Design review of the part built by this model. Coordinates are the model's own, in mm. A direction names the side the tool comes from. Coordinates: 2 decimals unless noted, no trailing zeros. Loops run counter-clockwise (first coordinate to the right, second up) from the corner with the lowest first, then second, coordinate; pieces in that order, holes last. Notation, with made-up numbers: (53, 17) - (73, 17) arc R26 ccw to (73, 36) - close; hole circle Ø3 at (12.25, 13.25). An arc over 180 degrees is marked (long way). Answer in a Markdown table with one row per item. Add a question column.
(1) The part is to be moulded in two halves that separate along Z. For faces 1 (the face through (-55.431, 283.334, 42.503)), 2 (the face through (63.5, 283, 0)), 3 (the face through (0, 292.1, 42)), say which applies: released by +Z, released by -Z, zero draft, split by the parting line, or undercut.
(2) We need section A-A, the plane x = 0. Give the number of separate pieces and of enclosed holes in the cut face, plus the area to 3 significant figures.
(3) To check wall thickness, follow L1, parallel to Y at x = -67.5, z = 0; L2, parallel to X at y = 163, z = 3; L3, parallel to Y at x = -31.5, z = -47. State the ranges of each line that lie inside material, in increasing order. Write a range as [from, to].
(4) Clearance check with flat-ended pins moving along their axes: pin 1 (1 mm diameter, centred on y = 231.5, z = 30, fed in from -X); pin 2 (5 mm diameter, centred on x = 59.92, z = 0, fed in from +Y); pin 3 (3 mm diameter, centred on x = -48, y = 205.5, fed in from -Z); pin 4 (4 mm diameter, centred on x = -22.93, z = -55.36, fed in from +Y). State where each tip first meets the part, or that it passes through.
(5) For faces 4 (the face through (-52, 274.32, -21)), 5 (the face through (-19.997, 288.343, 56.574)), 6 (the face through (-44.89, 283.09, -44.3)), 7 (the face through (-63.5, 283, 0)), 8 (the face through (46.2, 292.1, 20.4)), list the 3-axis set-ups (+Z, -Z, +X, -X, +Y, -Y) from which the entire face can be reached by the end or side of a thin tool; tool diameter is ignored.
(6) We need section C-C, the plane y = 179. Write out the cut boundary in (x, z) (3 decimals), plus the area to 3 significant figures.
from build123d import *

# Parameters (mm, degrees)
SKETCH2_R               = 50.8
SKETCH2_R_2             = 41.275
BASE_CYLINDER_DEPTH     = 292.1
SKETCH3_R               = 69.85
SKETCH3_R_2             = 41.275
AFT_FLANGE_DEPTH        = 17.78
SKETCH4_R               = 69.85
SKETCH4_R_2             = 41.275
FORWARD_FLANGE_DEPTH    = 17.78
SKETCH6_R               = 50.0761
SKETCH6_R_2             = 47.0027
O_RING_SLOT_1_DEPTH     = 1.9812
SKETCH7_R               = 50.0761
SKETCH7_R_2             = 47.0027
O_RING_SLOT_2_DEPTH     = 1.9812
SKETCH8_R               = 3.175
CUT_EXTRUDE4_DEPTH      = 1
CUT_EXTRUDE4_DEPTH_BACK = 293.1
FILLET1_R               = 4.7625
SKETCH9_R               = 3.175
CUT_EXTRUDE5_DEPTH      = 7.62
SKETCH10_R              = 3.175
CUT_EXTRUDE6_DEPTH      = 7.62
CUT_EXTRUDE7_REACH      = 286.48
SKETCH11_R              = 1.4097
CUT_EXTRUDE8_REACH      = 286.48
SKETCH12_R              = 1.4097
SKETCH13_R              = 2.3114
CUT_EXTRUDE10_DEPTH     = 6.35
SKETCH14_R              = 2.3114
CUT_EXTRUDE11_DEPTH     = 6.35
SKETCH17_R              = 69.85
CUT_EXTRUDE12_DEPTH     = 146.05


with BuildPart() as part:
    # Sketch2 → Base Cylinder (new body)
    with BuildSketch(Plane(origin=(0, 0, 0), x_dir=(1, 0, 0), z_dir=(0, 1, 0))):
        Circle(SKETCH2_R)
        Circle(SKETCH2_R_2, mode=Mode.SUBTRACT)
    extrude(amount=BASE_CYLINDER_DEPTH)

    # Sketch3 → Aft Flange (add)
    with BuildSketch(Plane.XZ):
        Circle(SKETCH3_R)
        Circle(SKETCH3_R_2, mode=Mode.SUBTRACT)
    extrude(amount=-AFT_FLANGE_DEPTH)

    # Sketch4 → Forward Flange (add)
    with BuildSketch(Plane(origin=(0, 292.1, 0), x_dir=(1, 0, 0), z_dir=(0, 1, 0))):
        Circle(SKETCH4_R)
        Circle(SKETCH4_R_2, mode=Mode.SUBTRACT)
    extrude(amount=-FORWARD_FLANGE_DEPTH)

    # Sketch6 → O-Ring Slot 1 (cut)
    with BuildSketch(Plane.XZ):
        Circle(SKETCH6_R)
        Circle(SKETCH6_R_2, mode=Mode.SUBTRACT)
    extrude(amount=-O_RING_SLOT_1_DEPTH, mode=Mode.SUBTRACT)

    # Sketch7 → O-Ring Slot 2 (cut)
    with BuildSketch(Plane(origin=(0, 292.1, 0), x_dir=(1, 0, 0), z_dir=(0, 1, 0))):
        Circle(SKETCH7_R)
        Circle(SKETCH7_R_2, mode=Mode.SUBTRACT)
    extrude(amount=-O_RING_SLOT_2_DEPTH, mode=Mode.SUBTRACT)

    # Sketch8 → Cut-Extrude4 (cut, two sides)
    with BuildSketch(Plane.XZ) as cut_extrude4_sk:
        with Locations((-59.9186, 0)):
            Circle(SKETCH8_R)
        with Locations((-42.368848379, 42.368848379)):
            Circle(SKETCH8_R)
        with Locations((0, 59.9186)):
            Circle(SKETCH8_R)
        with Locations((42.368848379, 42.368848379)):
            Circle(SKETCH8_R)
        with Locations((59.9186, 0)):
            Circle(SKETCH8_R)
        with Locations((42.368848379, -42.368848379)):
            Circle(SKETCH8_R)
        with Locations((0, -59.9186)):
            Circle(SKETCH8_R)
        with Locations((-42.368848379, -42.368848379)):
            Circle(SKETCH8_R)
    extrude(amount=CUT_EXTRUDE4_DEPTH, mode=Mode.SUBTRACT)
    extrude(cut_extrude4_sk.sketch, amount=-CUT_EXTRUDE4_DEPTH_BACK, mode=Mode.SUBTRACT)

    # Fillet1
    fillet1_edges = [part.edges().sort_by_distance(p)[0] for p in [
        (-50.8, 17.78, 0),
        (-50.8, 274.32, 0),
    ]]
    fillet(fillet1_edges, radius=FILLET1_R)

    # Sketch9 → Cut-Extrude5 (cut)
    with BuildSketch(Plane(origin=(0, 292.1, 0), x_dir=(1, 0, 0), z_dir=(0, 1, 0))):
        with Locations((-22.929855511, 55.357568157)):
            Circle(SKETCH9_R)
        with Locations((22.929855511, -55.357568157)):
            Circle(SKETCH9_R)
        with Locations((22.929855511, 55.357568157)):
            Circle(SKETCH9_R)
        with Locations((-22.929855511, -55.357568157)):
            Circle(SKETCH9_R)
    extrude(amount=-CUT_EXTRUDE5_DEPTH, mode=Mode.SUBTRACT)

    # Sketch10 → Cut-Extrude6 (cut)
    with BuildSketch(Plane.XZ):
        with Locations((-22.929855511, 55.357568157)):
            Circle(SKETCH10_R)
        with Locations((22.929855511, -55.357568157)):
            Circle(SKETCH10_R)
        with Locations((22.929855511, 55.357568157)):
            Circle(SKETCH10_R)
        with Locations((-22.929855511, -55.357568157)):
            Circle(SKETCH10_R)
    extrude(amount=-CUT_EXTRUDE6_DEPTH, mode=Mode.SUBTRACT)

    # Sketch11 → Cut-Extrude7 (cut, up to next)
    with BuildSketch(Plane(origin=(0, 284.48, 0), x_dir=(1, 0, 0), z_dir=(0, 1, 0)), mode=Mode.PRIVATE) as cut_extrude7_sk1:
        with Locations((-22.929855511, 55.357568157)):
            Circle(SKETCH11_R)
    cut_extrude7_tool1 = extrude(cut_extrude7_sk1.sketch, amount=-CUT_EXTRUDE7_REACH, mode=Mode.PRIVATE) & part.part
    add(cut_extrude7_tool1.solids().sort_by_distance((-22.929856, 284.48, -55.357568))[0], mode=Mode.SUBTRACT)
    # Sketch11 → Cut-Extrude7 (cut, up to next)
    with BuildSketch(Plane(origin=(0, 284.48, 0), x_dir=(1, 0, 0), z_dir=(0, 1, 0)), mode=Mode.PRIVATE) as cut_extrude7_sk2:
        with Locations((22.929855511, 55.357568157)):
            Circle(SKETCH11_R)
    cut_extrude7_tool2 = extrude(cut_extrude7_sk2.sketch, amount=-CUT_EXTRUDE7_REACH, mode=Mode.PRIVATE) & part.part
    add(cut_extrude7_tool2.solids().sort_by_distance((22.929856, 284.48, -55.357568))[0], mode=Mode.SUBTRACT)
    # Sketch11 → Cut-Extrude7 (cut, up to next)
    with BuildSketch(Plane(origin=(0, 284.48, 0), x_dir=(1, 0, 0), z_dir=(0, 1, 0)), mode=Mode.PRIVATE) as cut_extrude7_sk3:
        with Locations((-22.929855511, -55.357568157)):
            Circle(SKETCH11_R)
    cut_extrude7_tool3 = extrude(cut_extrude7_sk3.sketch, amount=-CUT_EXTRUDE7_REACH, mode=Mode.PRIVATE) & part.part
    add(cut_extrude7_tool3.solids().sort_by_distance((-22.929856, 284.48, 55.357568))[0], mode=Mode.SUBTRACT)
    # Sketch11 → Cut-Extrude7 (cut, up to next)
    with BuildSketch(Plane(origin=(0, 284.48, 0), x_dir=(1, 0, 0), z_dir=(0, 1, 0)), mode=Mode.PRIVATE) as cut_extrude7_sk4:
        with Locations((22.929855511, -55.357568157)):
            Circle(SKETCH11_R)
    cut_extrude7_tool4 = extrude(cut_extrude7_sk4.sketch, amount=-CUT_EXTRUDE7_REACH, mode=Mode.PRIVATE) & part.part
    add(cut_extrude7_tool4.solids().sort_by_distance((22.929856, 284.48, 55.357568))[0], mode=Mode.SUBTRACT)

    # Sketch12 → Cut-Extrude8 (cut, up to next)
    with BuildSketch(Plane.XZ.offset(-7.62), mode=Mode.PRIVATE) as cut_extrude8_sk1:
        with Locations((-22.929855511, 55.357568157)):
            Circle(SKETCH12_R)
    cut_extrude8_tool1 = extrude(cut_extrude8_sk1.sketch, amount=-CUT_EXTRUDE8_REACH, mode=Mode.PRIVATE) & part.part
    add(cut_extrude8_tool1.solids().sort_by_distance((-22.929856, 7.62, 55.357568))[0], mode=Mode.SUBTRACT)
    # Sketch12 → Cut-Extrude8 (cut, up to next)
    with BuildSketch(Plane.XZ.offset(-7.62), mode=Mode.PRIVATE) as cut_extrude8_sk2:
        with Locations((22.929855511, 55.357568157)):
            Circle(SKETCH12_R)
    cut_extrude8_tool2 = extrude(cut_extrude8_sk2.sketch, amount=-CUT_EXTRUDE8_REACH, mode=Mode.PRIVATE) & part.part
    add(cut_extrude8_tool2.solids().sort_by_distance((22.929856, 7.62, 55.357568))[0], mode=Mode.SUBTRACT)
    # Sketch12 → Cut-Extrude8 (cut, up to next)
    with BuildSketch(Plane.XZ.offset(-7.62), mode=Mode.PRIVATE) as cut_extrude8_sk3:
        with Locations((-22.929855511, -55.357568157)):
            Circle(SKETCH12_R)
    cut_extrude8_tool3 = extrude(cut_extrude8_sk3.sketch, amount=-CUT_EXTRUDE8_REACH, mode=Mode.PRIVATE) & part.part
    add(cut_extrude8_tool3.solids().sort_by_distance((-22.929856, 7.62, -55.357568))[0], mode=Mode.SUBTRACT)
    # Sketch12 → Cut-Extrude8 (cut, up to next)
    with BuildSketch(Plane.XZ.offset(-7.62), mode=Mode.PRIVATE) as cut_extrude8_sk4:
        with Locations((22.929855511, -55.357568157)):
            Circle(SKETCH12_R)
    cut_extrude8_tool4 = extrude(cut_extrude8_sk4.sketch, amount=-CUT_EXTRUDE8_REACH, mode=Mode.PRIVATE) & part.part
    add(cut_extrude8_tool4.solids().sort_by_distance((22.929856, 7.62, -55.357568))[0], mode=Mode.SUBTRACT)

    # Sketch13 → Cut-Extrude10 (cut)
    with BuildSketch(Plane(origin=(-69.85, 0, 0), x_dir=(0, 0, -1), z_dir=(1, 0, 0))):
        with Locations((0, 283.21)):
            Circle(SKETCH13_R)
    extrude(amount=CUT_EXTRUDE10_DEPTH, mode=Mode.SUBTRACT)

    # Sketch14 → Cut-Extrude11 (cut)
    with BuildSketch(Plane(origin=(69.85, 0, 0), x_dir=(0, 0, -1), z_dir=(1, 0, 0))):
        with Locations((0, 283.21)):
            Circle(SKETCH14_R)
    extrude(amount=-CUT_EXTRUDE11_DEPTH, mode=Mode.SUBTRACT)

    # Sketch17 → Cut-Extrude12 (cut)
    with BuildSketch(Plane(origin=(0, 0, 0), x_dir=(-1, 0, 0), z_dir=(0, -1, 0))):
        Circle(SKETCH17_R)
    extrude(amount=-CUT_EXTRUDE12_DEPTH, mode=Mode.SUBTRACT)


solid = part.part
Responses:
| question | item | result |
|---|---|---|
| 1 | face 1 | split by the parting line |
| 1 | face 2 | undercut |
| 1 | face 3 | zero draft |
| 2 | separate pieces | 4 |
| 2 | enclosed holes | 0 |
| 2 | area | 3,230 mm2 |
| 3 | L1 | y = [274.32, 280.9], [285.52, 292.1] |
| 3 | L2 | x = [-50.71, -41.17], [41.17, 50.71] |
| 3 | L3 | y = [274.32, 292.1] |
| 4 | pin 1 | stops at x = -41.36 |
| 4 | pin 2 | passes through |
| 4 | pin 3 | stops at z = -20.45 |
| 4 | pin 4 | stops at y = 284.48 |
| 5 | face 4 | -Y |
| 5 | face 5 | +Y |
| 5 | face 6 | +Y, -Y |
| 5 | face 7 | -X |
| 5 | face 8 | +Z, -Z, +X, -X, +Y |
| 6 | outline | circle Ø101.6 at (0, 0); hole circle Ø82.55 at (0, 0) |
| 6 | area | 2,760 mm2 |
